CAD build for the part. Positions are in the model's coordinates, mm. A direction names the side the tool comes from. Give positions to 0.01 mm unless a question says otherwise; leave off trailing zeros. Order: outer loops, then holes, each group sorted by start corner. A loop starts at its lowest first (then second) coordinate and runs counter-clockwise, first axis right, second up.
Item 1: Which spindle directions (+Z, -Z, +X, -X, +Y, -Y) get a long thin tool onto all of the face, cutting with end or side? Do faces 4 (the flat face through (25, 0, -8)), 5 (the flat face through (-3, -12, -6)). Say none if no direction does.
Item 2: Flat gauge pins, fed straight in: P1, Ø10, axis at x = -27, z = -19, coming from the +Y side; P2, Ø2, axis at y = -12, z = -29.5, coming from the +X side; P3, Ø4, axis at y = -22, z = -5, coming from the -X side; P4, Ø8, axis at x = 0.5, y = -39, coming from the -Z side. Where does each tip first touch, or does it go through?
Item 3: Band-saw the part on D-D on y = -8. Give the cut face in (x, z).
Item 4: Two-plate mould, pull along Z, no slides. Class faces 1 (the cylindrical face through (26.34, -24.79, 41.32)), 2 (the cylindrical face through (-5.158, -13.479, -3.955)), 3 (the flat face through (-1, -50, -8)): released by +Z, released by -Z, zero draft, split by the parting line, or undercut.
Item 5: Band-saw the part on C-C on y = -18.5. Give the cut face in (x, z), plus the area to 3 significant figures.
Item 6: Wall check: L1, parallel to Z at x = -18, y = -7.5; L2, parallel to Z at x = 0, y = -13.4; L3, parallel to X at y = -32.5, z = -37.5. Give the ranges that are in metal, low to high.
```python
from build123d import *

# Parameters (mm, degrees)
F0_R     = 49
F1_DEPTH = 50
F2_R     = 10
F4_R     = 25.5
F4_R_2   = 6.5
F5_DEPTH = 12
F6_DEPTH = 15
F7_R     = 11.99999
F4_R_3   = 3
F8_DEPTH = 50.001


# Not quite as in the source:
# - a fillet or chamfer is up to 0.001 mm smaller than in the source, because OpenCascade refuses the exact size


with BuildPart() as f1:
    # F0 (on Front) → F1 (new body)
    with BuildSketch(Plane.XZ):
        Circle(F0_R)
    extrude(amount=F1_DEPTH)

    # F2
    f2_edges = [f1.edges().sort_by_distance(p)[0] for p in [
        (-49, -50, 0),
        (-49, 0, 0),
    ]]
    fillet(f2_edges, radius=F2_R)

    # F4 (on Front) → F5 (cut)
    with BuildSketch(Plane.XZ):
        Circle(F4_R)
        Circle(F4_R_2, mode=Mode.SUBTRACT)
    extrude(amount=F5_DEPTH, mode=Mode.SUBTRACT)

    # F6 (cut): a face of the model
    f6_faces = [f1.faces().sort_by_distance(p)[0] for p in [
        (0, 0, 0),
    ]]
    extrude(f6_faces, amount=-F6_DEPTH, mode=Mode.SUBTRACT)

    # F7 (radius 12 in the source; OpenCascade refuses exactly that, so slightly less here)
    f7_edges = [f1.edges().sort_by_distance(p)[0] for p in [
        (-25.5, -12, 0),
    ]]
    fillet(f7_edges, radius=F7_R)

    # F4 (on Front) → F8 (cut, through all)
    with BuildSketch(Plane.XZ):
        Circle(F4_R_3)
    extrude(amount=F8_DEPTH, mode=Mode.SUBTRACT)


solid = f1.part
```
The answers:
1. face 4: +Z, -Z, +X, -X, +Y
1. face 5: +Y
2. P1: stops at y = 0
2. P2: stops at x = 39.86
2. P3: stops at x = -48.91
2. P4: stops at z = -49
3. outline: circle Ø97.6 at (0, 0); hole circle Ø44.89 at (0, 0)
4. face 1: split by the parting line
4. face 2: undercut
4. face 3: zero draft
5. outline: circle Ø98 at (0, 0); hole circle Ø6 at (0, 0)
5. area: 7,510 mm2
6. L1: z = -45.23 to -14.1, 14.1 to 45.23
6. L2: z = -49 to -6.5, 6.5 to 49
6. L3: x = -31.54 to 31.54
